from build123d import *

# Parameters (mm, degrees)
F0_W     = 44.45
F0_H     = 35
F1_DEPTH = 25
F2_T     = -7
F3_D     = 2
F3_DEPTH = 3
F3_TIP   = 0.600860619


with BuildPart() as f1:
    # F0 (on Front) → F1 (new body)
    with BuildSketch(Plane.XZ):
        with Locations((-22.225, 17.5)):
            Rectangle(F0_W, F0_H)
    extrude(amount=F1_DEPTH)

    # F2
    f2_openings = [f1.faces().sort_by_distance(p)[0] for p in [
        (-22.225, 0, 17.5),
    ]]
    offset(amount=F2_T, openings=f2_openings)

    # F3
    with Locations(Plane(origin=(0, 0, 0), x_dir=(1, 0, 0), z_dir=(0, 1, 0))):
        with Locations((-3.7769665942, -30.7552888989), (-40.1591621339, -30.7552888989), (-40.1591621339, -4.2394511402), (-3.7769665942, -4.2394511402)):
            Hole(F3_D / 2, depth=F3_DEPTH)
            with Locations((0, 0, -(F3_DEPTH + F3_TIP / 2))):  # 118° drill point
                Cone(0, F3_D / 2, F3_TIP, mode=Mode.SUBTRACT)


solid = f1.part
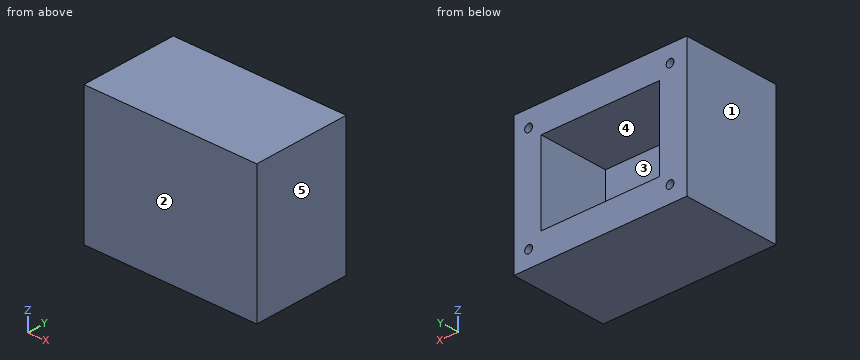
The model under review builds one solid part; all positions refer to its coordinate system, in mm. Face numbers are marked on the shaded views. A direction names the side the tool comes from. Give positions to 0.01 mm unless a question says otherwise; leave off trailing zeros. Write each loop counter-clockwise with the first axis right and the second up, starting at its lowest first coordinate (ties: lowest second). Pieces come first, ordered by that corner, then holes.
1. Add section C-C, the plane x = -34. Write out the cut boundary in (y, z), plus the area to 3 significant figures.
2. Add section B-B, the plane z = 26. Write out the cut boundary in (x, y), plus the area to 3 significant figures.
3. Add section A-A, the plane y = -15. Write out the cut boundary in (x, z).
4. Wall thickness on L1, parallel to X at y = -17.5, z = 13; L2, parallel to Z at x = -34.5, y = -14; L3, parallel to Y at x = -13, z = 23.5: over which ranges is each line inside the solid? List them lowest first.
5. Tool access review of the marked faces 4 and 5: name each direction out of +Z, -Z, +X, -X, +Y, -Y from which nothing blocks a thin tool from reaching the whole face with its end or side.
6. Draft analysis for pull direction X (two halves, no side actions). For the marked faces 1, 2 and 3, state which applies: +X half, -X half, draft (parallel to the pull), parting line (faces both ways), or undercut.
7. For P1, Ø1.2, axis at x = -3.78, z = 30.76, coming from the +Y side; P2, Ø17, axis at x = -27.5, z = 18.5, coming from the +Y side, all flat-tipped, find the tip position at first contact; note any pin that passes through.
Worked answers:
1. outline: (-25, 0) - (0, 0) - (0, 7) - (-18, 7) - (-18, 28) - (0, 28) - (0, 35) - (-25, 35) - close
1. area: 497 mm2
2. outline: (-44.45, -25) - (0, -25) - (0, 0) - (-7, 0) - (-7, -18) - (-37.45, -18) - (-37.45, 0) - (-44.45, 0) - close
2. area: 563 mm2
3. outline: (-44.45, 0) - (0, 0) - (0, 35) - (-44.45, 35) - close; hole (-37.45, 7) - (-7, 7) - (-7, 28) - (-37.45, 28) - close
4. L1: x = -44.45 to -37.45, -7 to 0
4. L2: z = 0 to 7, 28 to 35
4. L3: y = -25 to -18
5. face 4: +Y
5. face 5: +Z, -Z, +X, +Y, -Y
6. face 1: -X half
6. face 2: draft
6. face 3: undercut
7. P1: stops at y = -3.24
7. P2: stops at y = -18
